Source: three-view drawing plus pictorial views. Frame: mm from the lowest corner of the part. A direction names the side the tool comes from. Round coordinates to 2 decimals unless told otherwise and drop trailing zeros. Loops run counter-clockwise (first coordinate to the right, second up) from the corner with the lowest first, then second, coordinate; pieces in that order, holes last. Notation, with made-up numbers: (70.25, -20.5) -> (97.25, -20.5) arc R20 ccw to (97.25, 10.5) -> close; hole circle Ø5 at (12.5, 85.25). An arc over 180 degrees is marked (long way). Answer in a Markdown table with one row per item.
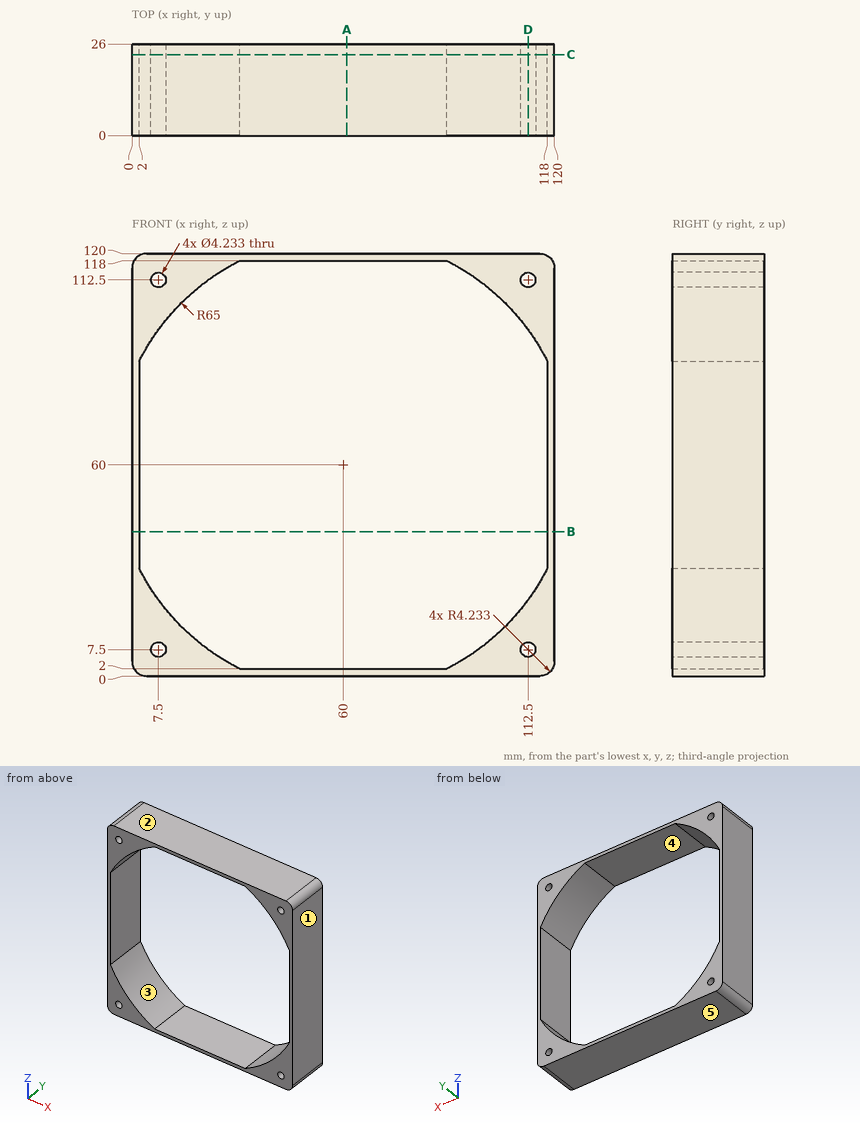
Item 1: Cut plane C-C (y = 23). Output: boundary loops of the cut face in (x, z), then the cut area to 3 significant figures.
Answer:
| item | result |
|---|---|
| outline | (0, 4.23) arc R4.23 ccw to (4.23, 0) -> (115.77, 0) arc R4.23 ccw to (120, 4.23) -> (120, 115.77) arc R4.23 ccw to (115.77, 120) -> (4.23, 120) arc R4.23 ccw to (0, 115.77) -> close; hole (2, 30.66) arc R65 ccw to (30.66, 2) -> (89.34, 2) arc R65 ccw to (118, 30.66) -> (118, 89.34) arc R65 ccw to (89.34, 118) -> (30.66, 118) arc R65 ccw to (2, 89.34) -> close; hole circle Ø4.23 at (7.5, 7.5); hole circle Ø4.23 at (7.5, 112.5); hole circle Ø4.23 at (112.5, 7.5); hole circle Ø4.23 at (112.5, 112.5) |
| area | 2,160 mm² |
Item 2: Pin query (flat end, axial travel): pin 1 Ø3.5 at (x, z) = (7.5, 7.5) entering from +Y. Return the tip coordinate at first contact, or that it passes through.
Answer:
| item | result |
|---|---|
| pin 1 | passes through |
Item 3: Line query: probe 1 along Z at (x, y) = (42.5, 16); probe 2 along Z at (x, y) = (111.5, 6) (1 decimal); probe 3 along X at (y, z) = (3.25, 113) (1 decimal). Output: solid intervals per line, ascending. Write a range as [from, to].
Answer:
| item | result |
|---|---|
| probe 1 | z = [0, 2], [118, 120] |
| probe 2 | z = [0, 5.6], [9.4, 20.3], [99.7, 110.6], [114.4, 120] |
| probe 3 | x = [0, 5.4], [9.6, 22.4], [97.6, 110.4], [114.6, 120] |
Item 4: Cut plane A-A (x = 61). Output: boundary loops of the cut face in (y, z).
Answer:
| item | result |
|---|---|
| outline | (0, 0) -> (26, 0) -> (26, 2) -> (0, 2) -> close; (0, 118) -> (26, 118) -> (26, 120) -> (0, 120) -> close |
Item 5: Cut plane D-D (x = 112.5). Output: boundary loops of the cut face in (y, z) (1 decimal).
Answer:
| item | result |
|---|---|
| outline | (0, 0) -> (26, 0) -> (26, 5.4) -> (0, 5.4) -> close; (0, 9.6) -> (26, 9.6) -> (26, 21.7) -> (0, 21.7) -> close; (0, 98.3) -> (26, 98.3) -> (26, 110.4) -> (0, 110.4) -> close; (0, 114.6) -> (26, 114.6) -> (26, 120) -> (0, 120) -> close |
Item 6: Cut plane B-B (z = 41). Output: boundary loops of the cut face in (x, y), then the cut area to 3 significant figures.
Answer:
| item | result |
|---|---|
| outline | (0, 0) -> (2, 0) -> (2, 26) -> (0, 26) -> close; (118, 0) -> (120, 0) -> (120, 26) -> (118, 26) -> close |
| area | 104 mm² |
Item 7: Reachability of the marked faces 4 and 5 from +Z, -Z, +X, -X, +Y, -Y: full face, straight path, thin tool, end or side. Return the list, or none.
Answer:
| item | result |
|---|---|
| face 4 | +Y, -Y |
| face 5 | -Z, +X, -X, +Y, -Y |
Item 8: Draft query along X for the marked faces 1, 2 and 3. Return one class per face: pulls with the +X half, pulls with the -X half, needs draft (parallel to the pull), parting line crosses it, or undercut.
Answer:
| item | result |
|---|---|
| face 1 | pulls with the +X half |
| face 2 | needs draft |
| face 3 | undercut |
